Input: dimensioned drawing with shaded views. Units: mm. Origin: part minimum x, y, z. A direction names the side the tool comes from. Give positions to 0.01 mm unless a question says otherwise; leave off trailing zeros. Write each loop counter-clockwise with the first axis right and the second up, starting at its lowest first coordinate (ties: lowest second). Pieces come first, ordered by that corner, then holes.
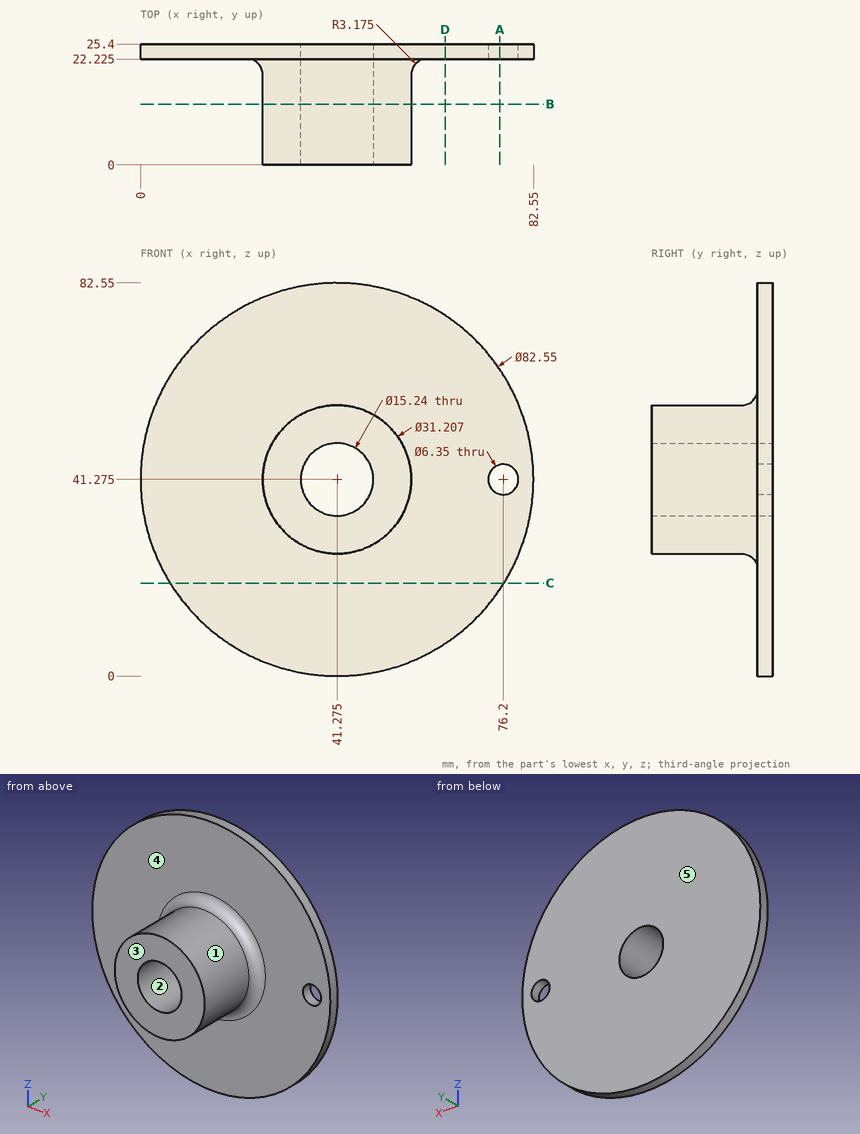
1. Cut plane C-C, the plane z = 19.5. Return the cut outline in (x, y) (1 decimal).
2. Line query: L1, parallel to Y at x = 16, z = 11 (1 decimal); L2, parallel to Z at x = 47, y = 18 (1 decimal); L3, parallel to X at y = 20.75, z = 47.5. Output: solid intervals per line, ascending.
3. Contact query for flat-ended pins moving along their axis: P1, Ø8, axis at y = 4, z = 56.5, coming from the +X side; P2, Ø10, axis at y = 14, z = 28.5, coming from the -X side; P3, Ø4, axis at x = 66, y = 19, coming from the +Z side; P4, Ø4, axis at y = 12, z = 51, coming from the +X side. Output: stop coordinate, or through.
4. Access query for the marked faces 4 and 5. Directions: +Z, -Z, +X, -X, +Y, -Y. A direction counts if a zero-diameter tool reaches every point of the face in a straight line with its end or side. Return the directions, or none.
5. Cut plane B-B, the plane y = 12.75. Return the cut outline in (x, z) (1 decimal).
6. Mould query, pull axis X, two halves, no side actions, for the marked faces 1, 2 and 3. Classes: +X half, -X half, draft (parallel to the pull), parting line (faces both ways), or undercut.
7. Cut plane A-A, the plane x = 75.5. Return the cut outline in (y, z) (1 decimal).
8. Cut plane D-D, the plane x = 64. Return the cut outline in (y, z) (1 decimal), then the cut area to 3 significant figures.
Response values:
1. outline: (6.2, 22.2) - (76.3, 22.2) - (76.3, 25.4) - (6.2, 25.4) - close
2. L1: y = 22.2 to 25.4
2. L2: z = 26.8 to 36.2, 46.3 to 55.8
2. L3: x = 26.43 to 36.88, 45.67 to 56.12
3. P1: stops at x = 52.11
3. P2: stops at x = 27.75
3. P3: passes through
3. P4: stops at x = 54.83
4. face 4: -Y
4. face 5: +Z, -Z, +X, -X, +Y
5. outline: circle Ø31.2 at (41.3, 41.3); hole circle Ø15.2 at (41.3, 41.3)
6. face 1: parting line
6. face 2: undercut
6. face 3: draft
7. outline: (22.2, 18.2) - (25.4, 18.2) - (25.4, 38.2) - (22.2, 38.2) - close; (22.2, 44.4) - (25.4, 44.4) - (25.4, 64.3) - (22.2, 64.3) - close
8. outline: (22.2, 6.8) - (25.4, 6.8) - (25.4, 75.7) - (22.2, 75.7) - close
8. area: 219 mm2
